from build123d import *

# Parameters (mm, degrees)
BOSS_EXTRUDE1_DEPTH = 10
SKETCH2_R           = 2
CUT_EXTRUDE1_DEPTH  = 34.166247904
SKETCH3_R           = 2
CUT_EXTRUDE2_DEPTH  = 33.015621187


with BuildPart() as part:
    # Sketch1 → Boss-Extrude1 (new body)
    with BuildSketch(Plane.XY):
        Polygon((10, 0), (20, 0), (20, -5), (30, -5), (30, -10), (0, -10), (0, -5), (10, -5), align=None)
    extrude(amount=BOSS_EXTRUDE1_DEPTH)

    # Sketch2 → Cut-Extrude1 (cut, through all)
    with BuildSketch(Plane(origin=(0, 0, 0), x_dir=(1, 0, 0), z_dir=(0, 1, 0))):
        with Locations(Location((15, -5, 0), (0, 0, 270))):
            Circle(SKETCH2_R)
    extrude(amount=-CUT_EXTRUDE1_DEPTH, mode=Mode.SUBTRACT)

    # Sketch3 → Cut-Extrude2 (cut, through all)
    with BuildSketch(Plane(origin=(0, -5, 0), x_dir=(1, 0, 0), z_dir=(0, 1, 0))):
        with Locations(Location((5, -5, 0), (0, 0, 180))):
            Circle(SKETCH3_R)
        with Locations(Location((25, -5, 0), (0, 0, 180))):
            Circle(SKETCH3_R)
    extrude(amount=-CUT_EXTRUDE2_DEPTH, mode=Mode.SUBTRACT)


solid = part.part
CAD build for the part. Positions are in the model's coordinates, mm. A direction names the side the tool comes from. Round coordinates to 2 decimals unless told otherwise and drop trailing zeros. Order: outer loops, then holes, each group sorted by start corner. A loop starts at its lowest first (then second) coordinate and runs counter-clockwise, first axis right, second up. Notation, with made-up numbers: M 24,-14.75 L 38,-14.75 A9 ccw 38,-8.75 Z; hole C 71,69.5 d9. An arc over 180 degrees is marked long. Use one line per item in the form item = value.
Q1. Saw through at A-A on x = 5. Give the cut face in (y, z), then the cut area to 3 significant figures.
Recorded:
outline = M -10,0 L -5,0 L -5,3 L -10,3 Z; M -10,7 L -5,7 L -5,10 L -10,10 Z
area = 30.0 mm^2
Q2. Saw through at D-D on z = 8. Give the cut face in (x, y).
Recorded:
outline = M 0,-10 L 30,-10 L 30,-5 L 20,-5 L 20,0 L 10,0 L 10,-5 L 0,-5 Z
Q3. Saw through at B-B on z = 5. Give the cut face in (x, y), then the cut area to 3 significant figures.
Recorded:
outline = M 0,-10 L 3,-10 L 3,-5 L 0,-5 Z; M 7,-10 L 13,-10 L 13,0 L 10,0 L 10,-5 L 7,-5 Z; M 17,-10 L 23,-10 L 23,-5 L 20,-5 L 20,0 L 17,0 Z; M 27,-10 L 30,-10 L 30,-5 L 27,-5 Z
area = 120 mm^2
Q4. Which spindle directions (+Z, -Z, +X, -X, +Y, -Y) get a long thin tool onto all of the face, cutting with end or side? Do faces 1 (the cylindrical face through (27, -7, 5)), 2 (the flat face through (10, -3, 5)), 3 (the flat face through (20, -2, 5)). Say none if no direction does.
Recorded:
face_1 = +Y, -Y
face_2 = +Z, -Z, -X, +Y
face_3 = +Z, -Z, +X, +Y
Q5. Two-plate mould, pull along Z, no slides. Class faces 4 (the cylindrical face through (6.474, -7.465, 6.352)), 5 (the flat face through (22.7, -5, 4.9)), 6 (the flat face through (15, -6, 10)), 7 (the flat face through (15, -6, 0)): +Z half, -Z half, draft (parallel to the pull), parting line (faces both ways), or undercut.
Recorded:
face_4 = undercut
face_5 = draft
face_6 = +Z half
face_7 = -Z half
Q6. Flat gauge pins, fed straight in: P1, Ø1, axis at y = -2.5, z = 7.5, coming from the +X side; P2, Ø5, axis at x = 25, z = 5, coming from the +Y side; P3, Ø2.5, axis at x = 5, z = 5, coming from the +Y side; P4, Ø1.5, axis at y = -2.5, z = 6, coming from the -X side. Where does each tip first touch, or does it go through?
Recorded:
P1 = 20
P2 = -5
P3 = through
P4 = 10
Q7. Saw through at C-C on y = -5.75. Give the cut face in (x, z).
Recorded:
outline = M 0,0 L 30,0 L 30,10 L 0,10 Z; hole C 5,5 d4; hole C 15,5 d4; hole C 25,5 d4
Q8. Probe L1, parallel to X at y = -3.75, z = 5; L2, parallel to X at y = -6.25, z = 4; L3, parallel to X at y = -3, z = 7.25. List the from-to ranges inside material, lowest first.
Recorded:
L1 = 10 to 13, 17 to 20
L2 = 0 to 3.27, 6.73 to 13.27, 16.73 to 23.27, 26.73 to 30
L3 = 10 to 20
